from build123d import *

# Parameters (mm, degrees)
SKETCH1_W           = 200
SKETCH1_H           = 25
BOSS_EXTRUDE1_DEPTH = 10
SKETCH4_W           = 25.5
SKETCH4_H           = 25.5
CUT_EXTRUDE2_DEPTH  = 10
SKETCH2_W           = 18.5
SKETCH2_H           = 8.5
SKETCH2_W_2         = 8.5
SKETCH2_H_2         = 18.5
BOSS_EXTRUDE3_DEPTH = 10
SKETCH3_W           = 13.1
SKETCH3_H           = 25
SKETCH3_W_2         = 25
SKETCH3_H_2         = 13.1
CUT_EXTRUDE3_DEPTH  = 10
SKETCH5_W           = 25.5
SKETCH5_H           = 3
CUT_EXTRUDE4_DEPTH  = 13


with BuildPart() as part:
    # Sketch1 → Boss-Extrude1 (new body)
    with BuildSketch(Plane.XY):
        with Locations((100, 12.5)):
            Rectangle(SKETCH1_W, SKETCH1_H)
    extrude(amount=BOSS_EXTRUDE1_DEPTH)

    # Sketch4 → Cut-Extrude2 (cut)
    with BuildSketch(Plane.XY.offset(10)):
        with Locations((100, 25)):
            Rectangle(SKETCH4_W, SKETCH4_H)
    extrude(amount=-CUT_EXTRUDE2_DEPTH, mode=Mode.SUBTRACT)

    # Sketch2 → Boss-Extrude3 (add)
    with BuildSketch(Plane.XY.offset(10)):
        with Locations((187.65, 7.65)):
            Rectangle(SKETCH2_W, SKETCH2_H)
        with Locations((17.35, 12.65)):
            Rectangle(SKETCH2_W_2, SKETCH2_H_2)
    extrude(amount=BOSS_EXTRUDE3_DEPTH)

    # Sketch3 → Cut-Extrude3 (cut)
    with BuildSketch(Plane.XY.offset(10)):
        with Locations((6.55, 12.5)):
            Rectangle(SKETCH3_W, SKETCH3_H)
        with Locations((187.5, 18.45)):
            Rectangle(SKETCH3_W_2, SKETCH3_H_2)
    extrude(amount=-CUT_EXTRUDE3_DEPTH, mode=Mode.SUBTRACT)

    # Sketch5 → Cut-Extrude4 (cut)
    with BuildSketch(Plane(origin=(0, 12.25, 0), x_dir=(1, 0, 0), z_dir=(0, 1, 0))):
        with Locations((100, -8.5)):
            Rectangle(SKETCH5_W, SKETCH5_H)
    extrude(amount=-CUT_EXTRUDE4_DEPTH, mode=Mode.SUBTRACT)


solid = part.part
Geometry: final body of the model. Coordinates: model frame, mm. A direction names the side the tool comes from. Coordinates: 2 decimals unless noted, no trailing zeros. Order: outer loops, then holes, each group sorted by start corner. A loop starts at its lowest first (then second) coordinate and runs counter-clockwise, first axis right, second up.
(1) Section query C-C (z = 5). Return the cut outline in (x, y).
(2) Material intervals for probe 1 along X at (y, z) = (7.5, 7.75); probe 2 along X at (y, z) = (8.75, 13.5); probe 3 along Z at (x, y) = (163.5, 2), sorted ascending.
(3) Section query A-A (y = 16.5). Return the cut outline in (x, z).
(4) Section query B-B (z = 14). Return the cut outline in (x, y).
(5) Draft query along X for faces 1 (the face through (17, 3.4, 15)), 2 (the face through (200, 6, 5)), 3 (the face through (146, 13, 10)), 4 (the face through (21.6, 13, 15)). Return one class per face: pulls with the +X half, pulls with the -X half, needs draft (parallel to the pull), parting line crosses it, or undercut.
(6) Section query D-D (y = 5.5). Return the cut outline in (x, z).
(7) First-contact query: pin 1 (3 mm diameter, centred on y = 20, z = 6.5, fed in from +X); pin 2 (10 mm diameter, centred on x = 104, y = 8.5, fed in from +Z); pin 3 (12.5 mm diameter, centred on x = 168.5, y = 8, fed in from +Z); pin 4 (12 mm diameter, centred on x = 172.5, z = 15.5, fed in from -Y). Flat tips, straight axial feed; report the tip coordinate or a pass-through.
(8) Access query for faces 5 (the face through (87.25, 15, 6)), 6 (the face through (100, 12.25, 4)), 7 (the face through (188, 3.4, 15)), 8 (the face through (187, 11.9, 10)). Directions: +Z, -Z, +X, -X, +Y, -Y. A direction counts if a zero-diameter tool reaches every point of the face in a straight line with its end or side. Return the directions, or none.
Solution:
1. outline: (13.1, 0) - (200, 0) - (200, 11.9) - (175, 11.9) - (175, 25) - (112.75, 25) - (112.75, 12.25) - (87.25, 12.25) - (87.25, 25) - (13.1, 25) - close
2. probe 1: x = 13.1 to 87.25, 112.75 to 200
2. probe 2: x = 13.1 to 21.6, 178.4 to 196.9
2. probe 3: z = 0 to 10
3. outline: (13.1, 0) - (87.25, 0) - (87.25, 10) - (21.6, 10) - (21.6, 20) - (13.1, 20) - close; (112.75, 0) - (175, 0) - (175, 10) - (112.75, 10) - close
4. outline: (13.1, 3.4) - (21.6, 3.4) - (21.6, 21.9) - (13.1, 21.9) - close; (178.4, 3.4) - (196.9, 3.4) - (196.9, 11.9) - (178.4, 11.9) - close
5. face 1: needs draft
5. face 2: pulls with the +X half
5. face 3: undercut
5. face 4: undercut
6. outline: (13.1, 0) - (200, 0) - (200, 10) - (196.9, 10) - (196.9, 20) - (178.4, 20) - (178.4, 10) - (112.75, 10) - (112.75, 7) - (87.25, 7) - (87.25, 10) - (21.6, 10) - (21.6, 20) - (13.1, 20) - close
7. pin 1: stops at x = 175
7. pin 2: stops at z = 7
7. pin 3: stops at z = 10
7. pin 4: stops at y = 0
8. face 5: +Z, +Y
8. face 6: +Z, -Z, +Y
8. face 7: +Z, +X, -X, -Y
8. face 8: +Z, -Z, +X, +Y
